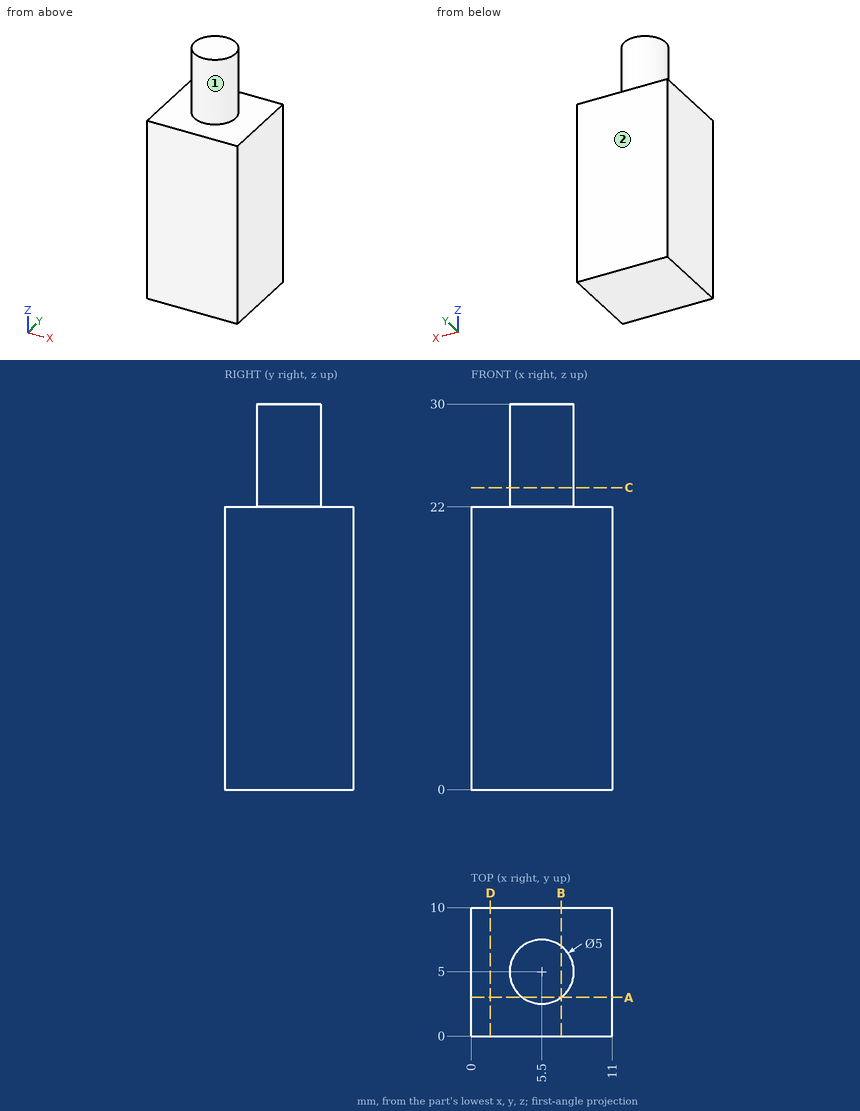
Part print with two shaded views. Sizes in mm from the minimum x, y, z corner. A direction names the side the tool comes from. Coordinates: 2 decimals unless noted, no trailing zeros. Loops run counter-clockwise (first coordinate to the right, second up) from the corner with the lowest first, then second, coordinate; pieces in that order, holes last. Notation, with made-up numbers: (-6.75, 7.5) - (12.25, 7.5) arc R26 cw to (12.25, 25.5) - close; hole circle Ø11 at (62.5, 87). An arc over 180 degrees is marked (long way). Write each question's results on one line, items separated by ' | '. Start each with the question number.
Q1. Slice it at B-B on x = 7. Give the cut face in (y, z).
Q2. Slice it at D-D on x = 1.5. Give the cut face in (y, z), and give its area (3 significant figures).
Q3. Which spindle directions (+Z, -Z, +X, -X, +Y, -Y) get a long thin tool onto all of the face, cutting with end or side? Do the marked faces 1 and 2. Say none if no direction does.
Q4. Probe line 1 along Z through (x, y) = (5, 9.5); line 2 along Y through (x, z) = (4, 28.5); line 3 along X through (y, z) = (5.5, 27.25). List the from-to ranges inside material, lowest first.
Q5. Slice it at C-C on z = 23.5. Give the cut face in (x, y), and give its area (3 significant figures).
Q6. Slice it at A-A on y = 3. Give the cut face in (x, z), and give its area (3 significant figures).
Q7. Drop a flat-ended pin along its axis: pin 1 Ø2 at (x, y) = (5, 1.5) entering from +Z. Give the stop position or say it passes through.
Answer:
1) outline: (0, 0) - (10, 0) - (10, 22) - (7, 22) - (7, 30) - (3, 30) - (3, 22) - (0, 22) - close
2) outline: (0, 0) - (10, 0) - (10, 22) - (0, 22) - close | area: 220 mm2
3) face 1: +Z | face 2: +Z, -Z, +X, -X, +Y
4) line 1: z = 0 to 22 | line 2: y = 3 to 7 | line 3: x = 3.05 to 7.95
5) outline: circle Ø5 at (5.5, 5) | area: 19.6 mm2
6) outline: (0, 0) - (11, 0) - (11, 22) - (7, 22) - (7, 30) - (4, 30) - (4, 22) - (0, 22) - close | area: 266 mm2
7) pin 1: stops at z = 22
